Source: CAD feature listing. Evaluate the final solid. Frame: model axes, mm. Face numbers are marked on the shaded views. A direction names the side the tool comes from. Round coordinates to 2 decimals unless told otherwise and drop trailing zeros. Write each loop counter-clockwise with the first axis right and the second up, starting at its lowest first coordinate (ties: lowest second). Pieces come first, ordered by that corner, then holes. Notation, with made-up numbers: (14, 57) -> (66, 57) arc R21 cw to (66, 81) -> close; hole circle Ø4 at (54, 11.5). An arc over 180 degrees is marked (long way). Put each result on its own line as item: value.
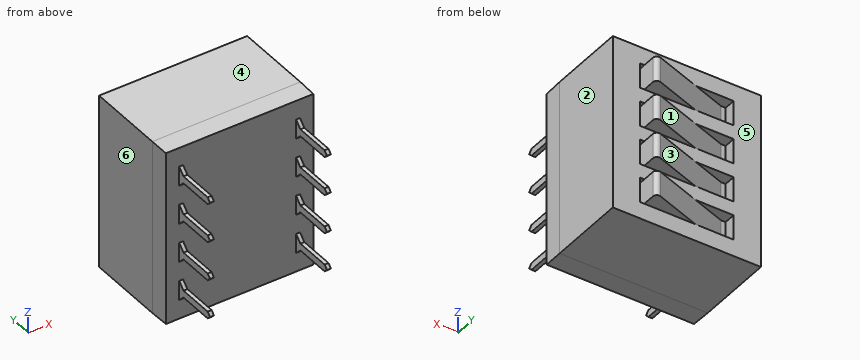
```python
from build123d import *

# Parameters (mm, degrees)
SKETCH1_W                = 11.43
SKETCH1_H                = 9.652
BASE_EXTRUDE_DEPTH       = 6.35
CHAMFER1_SIZE2           = 0.022167932
CHAMFER1_SIZE            = 1.27
BOSS_EXTRUDE_THIN1_DEPTH = 0.635
CUT_EXTRUDE1_DEPTH       = 2.143
CUT_EXTRUDE2_DEPTH       = 2.143
LPATTERN2_COUNT          = 4
LPATTERN2_PITCH          = 2.54
MIRROR1_COPY_1_DEPTH     = 0.635
MIRROR1_COPY_2_DEPTH     = 0.635
MIRROR1_COPY_3_DEPTH     = 0.635
MIRROR1_COPY_4_DEPTH     = 2.143
MIRROR1_COPY_5_DEPTH     = 2.143
MIRROR1_COPY_6_DEPTH     = 2.143
MIRROR1_COPY_7_DEPTH     = 2.143
MIRROR1_COPY_8_DEPTH     = 2.143
MIRROR1_COPY_9_DEPTH     = 2.143
SKETCH6_W                = 6.096
SKETCH6_H                = 1.6256
CUT_EXTRUDE3_DEPTH       = 0.762
BOSS_EXTRUDE1_DEPTH      = 1.6256
LPATTERN3_COUNT          = 4
LPATTERN3_PITCH          = 2.54


with BuildPart() as part:
    # Sketch1 → Base-Extrude (new body)
    with BuildSketch(Plane(origin=(0, 0.381, 0), x_dir=(0, 0, -1), z_dir=(0, 1, 0))):
        with Locations((-3.81, -3.81)):
            Rectangle(SKETCH1_W, SKETCH1_H)
    extrude(amount=BASE_EXTRUDE_DEPTH)

    # Chamfer1
    chamfer1_edges = [part.edges().sort_by_distance(p)[0] for p in [
        (8.636, 0.381, 3.81),
        (3.81, 0.381, 9.525),
        (-1.016, 0.381, 3.81),
        (3.81, 0.381, -1.905),
    ]]
    chamfer(chamfer1_edges, length=CHAMFER1_SIZE, length2=CHAMFER1_SIZE2)

    # Sketch3 → Boss-Extrude-Thin1 (add, symmetric)
    with BuildSketch(Plane(origin=(10.541, 0, 0), x_dir=(-1, 0, 0), z_dir=(0, 0, -1))):
        with BuildLine():
            Line((9.271, 1.8796), (10.033, 1.8796))
            ThreePointArc((10.033, 1.8796), (10.302407684, 1.768007684), (10.414, 1.4986))
            Line((10.414, 1.4986), (10.414, -2.5654))
            Line((10.414, -2.5654), (10.668, -2.5654))
            Line((10.668, -2.5654), (10.668, 1.4986))
            ThreePointArc((10.668, 1.4986), (10.482012806, 1.947612806), (10.033, 2.1336))
            Line((10.033, 2.1336), (9.271, 2.1336))
            Line((9.271, 2.1336), (9.271, 1.8796))
        make_face()
    boss_extrude_thin1 = extrude(amount=BOSS_EXTRUDE_THIN1_DEPTH, both=True)

    # Sketch4 → Cut-Extrude1 (cut, through all)
    with BuildSketch(Plane(origin=(0.127, 0, 0), x_dir=(0, 0, -1), z_dir=(1, 0, 0))):
        Polygon((0.635, -2.5654), (0, -2.5654), (0.2286, -2.3368), (0.2286, -0.0254), (0.635, 0.381), align=None)
    cut_extrude1 = extrude(amount=-CUT_EXTRUDE1_DEPTH, mode=Mode.SUBTRACT)

    # Sketch5 → Cut-Extrude2 (cut, through all)
    with BuildSketch(Plane(origin=(0.127, 0, 0), x_dir=(0, 0, -1), z_dir=(1, 0, 0))):
        Polygon((-0.635, 0.381), (-0.2286, -0.0254), (-0.2286, -2.3368), (0, -2.5654), (-0.635, -2.5654), align=None)
    cut_extrude2 = extrude(amount=-CUT_EXTRUDE2_DEPTH, mode=Mode.SUBTRACT)

    # LPattern2: Boss-Extrude-Thin1, Cut-Extrude1, Cut-Extrude2 ×4
    with Locations(*[(0, 0, i * LPATTERN2_PITCH) for i in range(1, LPATTERN2_COUNT)]):
        add(boss_extrude_thin1)
        add(cut_extrude1, mode=Mode.SUBTRACT)
        add(cut_extrude2, mode=Mode.SUBTRACT)

    # Mirror1: Boss-Extrude-Thin1, Cut-Extrude1, Cut-Extrude2 across plane
    add(boss_extrude_thin1.mirror(Plane.ZY.offset(-3.81)))
    add(cut_extrude1.mirror(Plane.ZY.offset(-3.81)), mode=Mode.SUBTRACT)
    add(cut_extrude2.mirror(Plane.ZY.offset(-3.81)), mode=Mode.SUBTRACT)

    # Mirror1 copy 1 sketch → Mirror1 copy 1 (add, symmetric)
    with BuildSketch(Plane(origin=(-2.921, 0, 2.54), x_dir=(1, 0, 0), z_dir=(0, 0, -1))):
        with BuildLine():
            Line((9.271, -1.8796), (10.033, -1.8796))
            ThreePointArc((10.033, -1.8796), (10.302407684, -1.768007684), (10.414, -1.4986))
            Line((10.414, -1.4986), (10.414, 2.5654))
            Line((10.414, 2.5654), (10.668, 2.5654))
            Line((10.668, 2.5654), (10.668, -1.4986))
            ThreePointArc((10.668, -1.4986), (10.482012806, -1.947612806), (10.033, -2.1336))
            Line((10.033, -2.1336), (9.271, -2.1336))
            Line((9.271, -2.1336), (9.271, -1.8796))
        make_face()
    extrude(amount=MIRROR1_COPY_1_DEPTH, both=True)

    # Mirror1 copy 2 sketch → Mirror1 copy 2 (add, symmetric)
    with BuildSketch(Plane(origin=(-2.921, 0, 5.08), x_dir=(1, 0, 0), z_dir=(0, 0, -1))):
        with BuildLine():
            Line((9.271, -1.8796), (10.033, -1.8796))
            ThreePointArc((10.033, -1.8796), (10.302407684, -1.768007684), (10.414, -1.4986))
            Line((10.414, -1.4986), (10.414, 2.5654))
            Line((10.414, 2.5654), (10.668, 2.5654))
            Line((10.668, 2.5654), (10.668, -1.4986))
            ThreePointArc((10.668, -1.4986), (10.482012806, -1.947612806), (10.033, -2.1336))
            Line((10.033, -2.1336), (9.271, -2.1336))
            Line((9.271, -2.1336), (9.271, -1.8796))
        make_face()
    extrude(amount=MIRROR1_COPY_2_DEPTH, both=True)

    # Mirror1 copy 3 sketch → Mirror1 copy 3 (add, symmetric)
    with BuildSketch(Plane(origin=(-2.921, 0, 7.62), x_dir=(1, 0, 0), z_dir=(0, 0, -1))):
        with BuildLine():
            Line((9.271, -1.8796), (10.033, -1.8796))
            ThreePointArc((10.033, -1.8796), (10.302407684, -1.768007684), (10.414, -1.4986))
            Line((10.414, -1.4986), (10.414, 2.5654))
            Line((10.414, 2.5654), (10.668, 2.5654))
            Line((10.668, 2.5654), (10.668, -1.4986))
            ThreePointArc((10.668, -1.4986), (10.482012806, -1.947612806), (10.033, -2.1336))
            Line((10.033, -2.1336), (9.271, -2.1336))
            Line((9.271, -2.1336), (9.271, -1.8796))
        make_face()
    extrude(amount=MIRROR1_COPY_3_DEPTH, both=True)

    # Mirror1 copy 4 sketch → Mirror1 copy 4 (cut, through all)
    with BuildSketch(Plane(origin=(7.493, 0, 2.54), x_dir=(0, 0, -1), z_dir=(-1, 0, 0))):
        Polygon((0.635, 2.5654), (0, 2.5654), (0.2286, 2.3368), (0.2286, 0.0254), (0.635, -0.381), align=None)
    extrude(amount=-MIRROR1_COPY_4_DEPTH, mode=Mode.SUBTRACT)

    # Mirror1 copy 5 sketch → Mirror1 copy 5 (cut, through all)
    with BuildSketch(Plane(origin=(7.493, 0, 5.08), x_dir=(0, 0, -1), z_dir=(-1, 0, 0))):
        Polygon((0.635, 2.5654), (0, 2.5654), (0.2286, 2.3368), (0.2286, 0.0254), (0.635, -0.381), align=None)
    extrude(amount=-MIRROR1_COPY_5_DEPTH, mode=Mode.SUBTRACT)

    # Mirror1 copy 6 sketch → Mirror1 copy 6 (cut, through all)
    with BuildSketch(Plane(origin=(7.493, 0, 7.62), x_dir=(0, 0, -1), z_dir=(-1, 0, 0))):
        Polygon((0.635, 2.5654), (0, 2.5654), (0.2286, 2.3368), (0.2286, 0.0254), (0.635, -0.381), align=None)
    extrude(amount=-MIRROR1_COPY_6_DEPTH, mode=Mode.SUBTRACT)

    # Mirror1 copy 7 sketch → Mirror1 copy 7 (cut, through all)
    with BuildSketch(Plane(origin=(7.493, 0, 2.54), x_dir=(0, 0, -1), z_dir=(-1, 0, 0))):
        Polygon((-0.635, -0.381), (-0.2286, 0.0254), (-0.2286, 2.3368), (0, 2.5654), (-0.635, 2.5654), align=None)
    extrude(amount=-MIRROR1_COPY_7_DEPTH, mode=Mode.SUBTRACT)

    # Mirror1 copy 8 sketch → Mirror1 copy 8 (cut, through all)
    with BuildSketch(Plane(origin=(7.493, 0, 5.08), x_dir=(0, 0, -1), z_dir=(-1, 0, 0))):
        Polygon((-0.635, -0.381), (-0.2286, 0.0254), (-0.2286, 2.3368), (0, 2.5654), (-0.635, 2.5654), align=None)
    extrude(amount=-MIRROR1_COPY_8_DEPTH, mode=Mode.SUBTRACT)

    # Mirror1 copy 9 sketch → Mirror1 copy 9 (cut, through all)
    with BuildSketch(Plane(origin=(7.493, 0, 7.62), x_dir=(0, 0, -1), z_dir=(-1, 0, 0))):
        Polygon((-0.635, -0.381), (-0.2286, 0.0254), (-0.2286, 2.3368), (0, 2.5654), (-0.635, 2.5654), align=None)
    extrude(amount=-MIRROR1_COPY_9_DEPTH, mode=Mode.SUBTRACT)

    # Sketch6 → Cut-Extrude3 (cut)
    with BuildSketch(Plane(origin=(0, 6.731, 0), x_dir=(-1, 0, 0), z_dir=(0, 1, 0))):
        with Locations((-3.81, 0)):
            Rectangle(SKETCH6_W, SKETCH6_H)
    cut_extrude3 = extrude(amount=-CUT_EXTRUDE3_DEPTH, mode=Mode.SUBTRACT)

    # Sketch7 → Boss-Extrude1 (add)
    with BuildSketch(Plane.XY.offset(-0.8128)):
        with BuildLine():
            Line((1.062579803, 5.969), (6.240649344, 7.782334164))
            ThreePointArc((6.240649344, 7.782334164), (6.471556683, 7.749779505), (6.5786, 7.542608722))
            Line((6.5786, 7.542608722), (6.5786, 5.969))
            Line((6.5786, 5.969), (1.062579803, 5.969))
        make_face()
    boss_extrude1 = extrude(amount=BOSS_EXTRUDE1_DEPTH)

    # LPattern3: Cut-Extrude3, Boss-Extrude1 ×4
    with Locations(*[(0, 0, i * LPATTERN3_PITCH) for i in range(1, LPATTERN3_COUNT)]):
        add(cut_extrude3, mode=Mode.SUBTRACT)
        add(boss_extrude1)


solid = part.part
```
Q1. Reachability of the marked faces 5 and 6 from +Z, -Z, +X, -X, +Y, -Y: full face, straight path, thin tool, end or side. Return the list, or none.
Ans:
face 5: +Y
face 6: +Z, -Z, -X, +Y, -Y
Q2. Pin query (flat end, axial travel): pin 1 (0.9 mm diameter, centred on x = 4.5, y = 7.5, fed in from -Z); pin 2 (0.8 mm diameter, centred on y = 7, z = 7.5, fed in from +X); pin 3 (0.5 mm diameter, centred on x = 4.5, y = 7.5, fed in from -Z); pin 4 (4 mm diameter, centred on x = 3, z = 4.5, fed in from -Y). Return the tip coordinate at first contact, or that it passes through.
Ans:
pin 1: stops at z = -0.81
pin 2: stops at x = 8.64
pin 3: passes through
pin 4: stops at y = 0.38
Q3. Cut plane B-B on z = 3.5. Output: boundary loops of the cut face in (x, y), and give its area (3 significant figures).
Ans:
outline: (-1.02, 1.65) -> (-0.99, 0.38) -> (8.61, 0.38) -> (8.64, 1.65) -> (8.64, 6.73) -> (-1.02, 6.73) -> close
area: 61.3 mm^2
Q4. Cut plane A-A on x = 0.5. Output: boundary loops of the cut face in (y, z) (3 decimals).
Ans:
outline: (0.381, -1.883) -> (1.651, -1.905) -> (6.731, -1.905) -> (6.731, 9.525) -> (1.651, 9.525) -> (0.381, 9.503) -> close
Q5. Material intervals for line 1 (Y direction, x = 1.5, z = 3.75); line 2 (Y direction, x = 6.75, z = 5.25); line 3 (Z direction, x = 7.75, y = 1.25), sorted ascending. Write a range as [from, to].
Ans:
line 1: y = [0.38, 6.73]
line 2: y = [0.38, 5.97]
line 3: z = [-1.9, 9.52]
Q6. Cut plane C-C on x = 4.75. Output: boundary loops of the cut face in (y, z) (3 decimals), and give its area (3 significant figures).
Ans:
outline: (0.381, -1.883) -> (1.651, -1.905) -> (6.731, -1.905) -> (6.731, -0.813) -> (7.26, -0.813) -> (7.26, 0.813) -> (6.731, 0.813) -> (6.731, 1.727) -> (7.26, 1.727) -> (7.26, 3.353) -> (6.731, 3.353) -> (6.731, 4.267) -> (7.26, 4.267) -> (7.26, 5.893) -> (6.731, 5.893) -> (6.731, 6.807) -> (7.26, 6.807) -> (7.26, 8.433) -> (6.731, 8.433) -> (6.731, 9.525) -> (1.651, 9.525) -> (0.381, 9.503) -> close
area: 76.0 mm^2
Q7. Draft query along Z for the marked faces 1, 2, 3 and 4. Return one class per face: +Z half, -Z half, draft (parallel to the pull), parting line (faces both ways), or undercut.
Ans:
face 1: undercut
face 2: draft
face 3: undercut
face 4: +Z half
Q8. Cut plane D-D on y = 6.5. Give the number of separate pieces and of enclosed holes in the cut face, and give its area (3 significant figures).
Ans:
separate pieces: 1
enclosed holes: 8
area: 96.7 mm^2
